The listing builds one solid part. Answer for the finished solid, in the listing's coordinates (mm). A direction names the side the tool comes from. Coordinates: 2 decimals unless noted, no trailing zeros. Order: outer loops, then holes, each group sorted by start corner. A loop starts at its lowest first (then second) coordinate and runs counter-clockwise, first axis right, second up. Notation, with made-up numbers: (13.5, -7) - (46.5, -7) arc R15 cw to (46.5, 11) - close; hole circle Ø8 at (76.5, -28.75). An arc over 180 degrees is marked (long way). Use a Markdown table: item, result. Add a question column.
Item 1: The part is cut by section D-D, the plane z = -0.7. Give the vertices of the cut face in (x, y).
Item 2: Find the intervals of material crossed by line 1 along X through (y, z) = (-3, -2.7); line 2 along Z through (x, y) = (-126.25, -5); line 3 along Z through (x, y) = (-128, -0.75), in increasing order.
Item 3: Flat-ended cylindrical pins translate along their axes: P1, Ø1, axis at y = -3.5, z = 0, coming from the -X side; P2, Ø1.5, axis at x = -128.5, y = -4.5, coming from the +Z side. Find the tip coordinate at first contact, or state that the pin passes through.
Item 4: The part is cut by section C-C, the plane z = -2. Give the vertices of the cut face in (x, y).
Item 5: The part is cut by section B-B, the plane x = -126.05. Give the vertices of the cut face in (y, z) (3 decimals).
Item 6: For faces 1 (the flat face through (-124.6, -5.2, -1)), 2 (the cylindrical face through (-128.48, -0.82, -0.49)), 3 (the cylindrical face through (-124.31, -2.5, 0.64)), determine the directions among +Z, -Z, +X, -X, +Y, -Y from which every point of the face is accessible in a straight line to the end or side of a thin tool.
Item 7: The part is cut by section A-A, the plane y = -3.05. Give the vertices of the cut face in (x, z) (3 decimals), then the cut area to 3 significant figures.
from build123d import *

# Parameters (mm, degrees)
SKETCH1_R           = 3.3
BOSS_EXTRUDE2_DEPTH = 1
SKETCH4_R           = 2.25
BOSS_EXTRUDE3_DEPTH = 2
CHAMFER4_SIZE       = 0.25
SKETCH5_R           = 1.825
BOSS_EXTRUDE4_DEPTH = 1.3


with BuildPart() as part:
    # Sketch1 → Boss-Extrude2 (new body)
    with BuildSketch(Plane.XY):
        with Locations((-126.049999999, -3.05)):
            Circle(SKETCH1_R)
    extrude(amount=-BOSS_EXTRUDE2_DEPTH)

    # Sketch4 → Boss-Extrude3 (add)
    with BuildSketch(Plane(origin=(0, 0, -1), x_dir=(-1, 0, 0), z_dir=(0, 0, -1))):
        with Locations((126.049999999, -3.05)):
            Circle(SKETCH4_R)
    extrude(amount=BOSS_EXTRUDE3_DEPTH)

    # Chamfer4
    chamfer4_edges = [part.edges().sort_by_distance(p)[0] for p in [
        (-123.799999999, -3.05, -3),
    ]]
    chamfer(chamfer4_edges, length=CHAMFER4_SIZE)

    # Sketch5 → Boss-Extrude4 (add)
    with BuildSketch(Plane.XY):
        with Locations((-126.049999999, -3.05)):
            Circle(SKETCH5_R)
    extrude(amount=BOSS_EXTRUDE4_DEPTH)


solid = part.part
Solution:
| question | item | result |
|---|---|---|
| 1 | outline | circle Ø6.6 at (-126.05, -3.05) |
| 2 | line 1 | x = -128.3 to -123.8 |
| 2 | line 2 | z = -3 to 0 |
| 2 | line 3 | z = -1 to 0 |
| 3 | P1 | stops at x = -129.35 |
| 3 | P2 | stops at z = 0 |
| 4 | outline | circle Ø4.5 at (-126.05, -3.05) |
| 5 | outline | (-6.35, -1) - (-5.3, -1) - (-5.3, -2.75) - (-5.05, -3) - (-1.05, -3) - (-0.8, -2.75) - (-0.8, -1) - (0.25, -1) - (0.25, 0) - (-1.225, 0) - (-1.225, 1.3) - (-4.875, 1.3) - (-4.875, 0) - (-6.35, 0) - close |
| 6 | face 1 | -Z |
| 6 | face 2 | +Z, -Z |
| 6 | face 3 | +Z |
| 7 | outline | (-129.35, -1) - (-128.3, -1) - (-128.3, -2.75) - (-128.05, -3) - (-124.05, -3) - (-123.8, -2.75) - (-123.8, -1) - (-122.75, -1) - (-122.75, 0) - (-124.225, 0) - (-124.225, 1.3) - (-127.875, 1.3) - (-127.875, 0) - (-129.35, 0) - close |
| 7 | area | 20.3 mm2 |
